Part model, mm, in its own coordinate system. A direction names the side the tool comes from. Give positions to 0.01 mm unless a question says otherwise; leave off trailing zeros. Write each loop counter-clockwise with the first axis right and the second up, starting at its lowest first coordinate (ties: lowest second). Pieces come first, ordered by that corner, then holes. Notation, with made-up numbers: M 29.25,-38.5 L 70.25,-38.5 A25 ccw 70.25,-18.5 Z; hole C 7.5,83 d11. An arc over 180 degrees is marked long. Answer as CSV lines item,"result". Start each with the question number.
1) Wall check: line 1 along Y through (x, z) = (-12.7, 4.5) (3 decimals); line 2 along Z through (x, y) = (-14, -25); line 3 along X through (y, z) = (-12, 8). Give the ranges that are in metal, low to high. Write a range as from..to.
2) Mould opens along X. For faces 1 (the flat face through (-57, -63.5, 120)), 2 (the flat face through (-25.4, -13, 82)), 3 (the flat face through (-99, -15, 10.16)), 4 (the flat face through (-114.3, -13, 6)) say: pulls with the +X half, pulls with the -X half, needs draft (parallel to the pull), parting line crosses it, or undercut.
3) Tool access for faces 5 (the cylindrical face through (-10.18, -14.63, 5.01)), 6 (the cylindrical face through (-7.42, -14.89, 11.45)), 7 (the flat face through (-10, -7, 12.7)), 8 (the flat face through (-96, -10, 12.7)), 9 (the flat face through (-58, 0, 77)): list every direction of +Z, -Z, +X, -X, +Y, -Y with a clear straight run to the whole face (end or side of a thin tool).
4) Slice it at D-D, the plane y = -49. Give the cut face in (x, z) (3 decimals).
5) Slice it at C-C, the plane z = 18. Give the cut face in (x, y).
6) Slice it at A-A, the plane y = -12.7. Give the cut face in (x, z) (3 decimals), plus the area to 3 significant figures.
7) Pin check, flat tips, straight feed: pin 1 Ø1.5 at (x, y) = (-23.5, -10.5) entering from +Z; pin 2 Ø12.5 at (y, z) = (-16.5, 67.5) entering from -X; pin 3 Ø5.5 at (x, y) = (-13.5, -14.5) entering from +Z. Stop position of each tip, or through.
8) Slice it at B-B, the plane x = -101.6. Give the cut face in (y, z) (3 decimals).
```python
from build123d import *

# Parameters (mm, degrees)
F1_DEPTH       = 25.4
F3_DEPTH       = 38.1
F5_D           = 6.35
F5_CBORE_D     = 11.43
F5_CBORE_DEPTH = 2.54


with BuildPart() as f1:
    # F0 (on Front) → F1 (new body)
    with BuildSketch(Plane.XZ):
        Polygon((-114.3, 0), (0, 0), (0, 12.7), (-25.4, 12.7), (-25.4, 152.4), (-88.9, 152.4), (-88.9, 12.7), (-114.3, 12.7), align=None)
    extrude(amount=F1_DEPTH)

    # F2 (on face) → F3 (join)
    with BuildSketch(Plane.XZ.offset(25.4)):
        with BuildLine():
            ThreePointArc((-51.435, 119.6848), (-53.108885, 123.725915), (-57.15, 125.3998))
            ThreePointArc((-57.15, 125.3998), (-61.191115, 115.643685), (-51.435, 119.6848))
        make_face()
    extrude(amount=F3_DEPTH)

    # F5 (through all)
    with Locations(Plane.XY.offset(12.7)):
        with Locations((-101.6, -12.7), (-12.7, -12.7)):
            CounterBoreHole(F5_D / 2, F5_CBORE_D / 2, F5_CBORE_DEPTH)


solid = f1.part
```
Found:
1,line 1,"-25.4..-15.875, -9.525..0"
1,line 2,"0..12.7"
1,line 3,"-114.3..-104.7, -98.5..-15.8, -9.6..0"
2,face 1,"needs draft"
2,face 2,"pulls with the +X half"
2,face 3,"undercut"
2,face 4,"pulls with the -X half"
3,face 5,"+Z, -Z"
3,face 6,"+Z"
3,face 7,"+Z, +X, +Y, -Y"
3,face 8,"+Z, -X, +Y, -Y"
3,face 9,"+Z, -Z, +X, -X, +Y"
4,outline,"M -57.15,125.4 A5.715 ccw long -51.435,119.685 A5.715 ccw Z"
5,outline,"M -88.9,-25.4 L -25.4,-25.4 L -25.4,0 L -88.9,0 Z"
6,outline,"M -114.3,0 L -104.775,0 L -104.775,10.16 L -107.315,10.16 L -107.315,12.7 L -114.3,12.7 Z; M -98.425,0 L -15.875,0 L -15.875,10.16 L -18.415,10.16 L -18.415,12.7 L -25.4,12.7 L -25.4,152.4 L -88.9,152.4 L -88.9,12.7 L -95.885,12.7 L -95.885,10.16 L -98.425,10.16 Z; M -9.525,0 L 0,0 L 0,12.7 L -6.985,12.7 L -6.985,10.16 L -9.525,10.16 Z"
6,area,"10,100 mm²"
7,pin 1,"z = 12.7"
7,pin 2,"x = -88.9"
7,pin 3,"z = 10.16"
8,outline,"M -25.4,0 L -15.875,0 L -15.875,10.16 L -18.415,10.16 L -18.415,12.7 L -25.4,12.7 Z; M -9.525,0 L 0,0 L 0,12.7 L -6.985,12.7 L -6.985,10.16 L -9.525,10.16 Z"
